The figure shows three views and two pictorial views of one solid part (mm, origin at its lowest corner). Answer the questions. Give positions to 0.01 mm unless a question says otherwise; leave off trailing zeros. Loops run counter-clockwise (first coordinate to the right, second up) from the corner with the lowest first, then second, coordinate; pieces in that order, holes last. Notation, with made-up numbers: (78, -16) - (84, -16) arc R31 ccw to (84, 13) - close; hole circle Ø10 at (52.25, -17). An arc over 180 degrees is marked (long way). Use a Markdown table: item, result. Add a question column.
Item 1: Each of these flat-tipped pins is pushed along its axis until it touches: P1, Ø6, axis at x = 6.5, z = 34.5, coming from the +Y side; P2, Ø1.5, axis at x = 23, y = 16, coming from the +Z side (1 decimal); P3, Ø8, axis at x = 30.5, y = 32.5, coming from the -Z side. Where does it stop, or does it pass through?
Item 2: A cutting plane is placed at A-A (z = 43). Determine the outline of the cut face in (x, y) (1 decimal).
Item 3: For a pull along Z with two mould halves and no side action, classify the marked faces 1, 2 and 3 as +Z half, -Z half, draft (parallel to the pull), parting line (faces both ways), or undercut.
Item 4: A cutting plane is placed at B-B (y = 43). Determine the outline of the cut face in (x, z) (1 decimal).
Item 5: A cutting plane is placed at D-D (x = 19). Determine the outline of the cut face in (y, z) (1 decimal).
Item 6: A cutting plane is placed at C-C (x = 7.5). Determine the outline of the cut face in (y, z).
Item 7: Consider probe 1 along Y at (x, z) = (34.5, 13); probe 2 along Y at (x, z) = (3, 62.5); probe 3 along Z at (x, y) = (30.5, 26) (1 decimal). Determine where each line is inside the solid, lowest interval first. Write a range as [from, to].
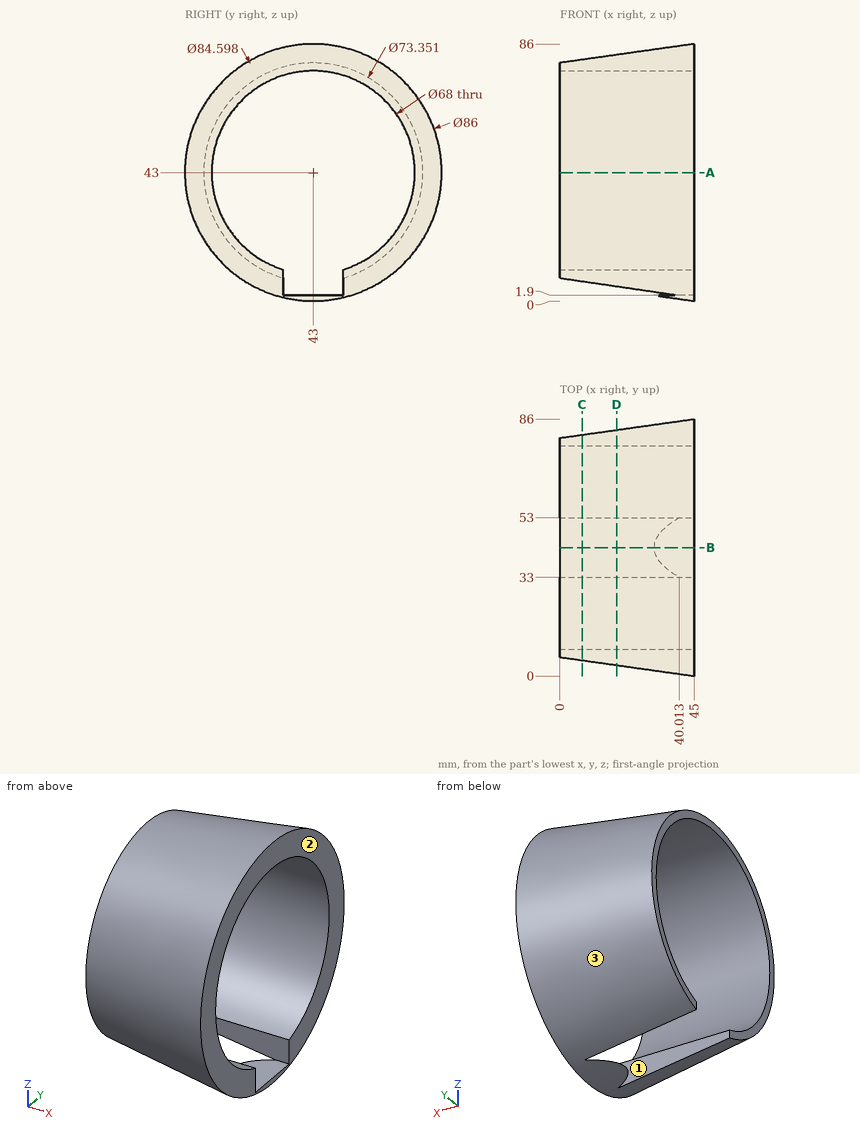
Geometry says:
| question | item | result |
|---|---|---|
| 1 | P1 | y = 80.35 |
| 1 | P2 | z = 73.1 |
| 1 | P3 | z = 2.7 |
| 2 | outline | (0, 6.3) - (45, 0) - (45, 9) - (0, 9) - close; (0, 77) - (45, 77) - (45, 86) - (0, 79.7) - close |
| 3 | face 1 | undercut |
| 3 | face 2 | draft |
| 3 | face 3 | parting line |
| 4 | outline | (0, 77) - (45, 77) - (45, 86) - (0, 79.7) - close; (31.5, 1.9) - (45, 0) - (45, 1.9) - close |
| 5 | outline | (33, 4.9) - (33, 10.5) arc R34 cw (long way) to (53, 10.5) - (53, 4.9) arc R39.3 ccw (long way) to start |
| 6 | outline | (33, 6.62) - (33, 10.5) arc R34 cw (long way) to (53, 10.5) - (53, 6.62) arc R37.73 ccw (long way) to start |
| 7 | probe 1 | [14.29, 27], [59, 71.71] |
| 7 | probe 2 | [11.44, 15.15], [70.85, 74.56] |
| 7 | probe 3 | [5.7, 13.6], [72.4, 80.3] |
